Design review of the part built by this model. Coordinates are the model's own, in mm. A direction names the side the tool comes from. Round coordinates to 2 decimals unless told otherwise and drop trailing zeros. Order: outer loops, then holes, each group sorted by start corner. A loop starts at its lowest first (then second) coordinate and runs counter-clockwise, first axis right, second up. Notation, with made-up numbers: (16, 14.5) - (33, 14.5) arc R31 ccw to (33, 46.5) - close; hole circle Ø2 at (33, -15.75). An arc over 180 degrees is marked (long way). Use CSV: the item, a comma, the result in double quotes.
from build123d import *

# Parameters (mm, degrees)
SKETCH1_W              = 200
SKETCH1_H              = 140
BOSS_EXTRUDE1_DEPTH    = 6.35
SKETCH4_W              = 65
SKETCH4_H              = 6.35
BOSS_EXTRUDE2_DEPTH    = 6.35
LPATTERN1_COUNT        = 2
LPATTERN1_PITCH        = 85
SKETCH5_W              = 6.35
SKETCH5_H              = 65
BOSS_EXTRUDE3_DEPTH    = 6.35
SKETCH6_W              = 65
SKETCH6_H              = 6.35
CUT_EXTRUDE3_DEPTH     = 6.35
SKETCH7_R              = 2
CUT_EXTRUDE4_DEPTH     = 6.35
FILLET4_R              = 1
LPATTERN2_COUNT        = 2
LPATTERN2_PITCH        = 85
FILLET4_OF_LPATTERN2_R = 1
FILLET5_R              = 5
SKETCH8_R              = 2
CUT_EXTRUDE6_DEPTH     = 6.35
FILLET6_R              = 1


with BuildPart() as part:
    # Sketch1 → Boss-Extrude1 (new body)
    with BuildSketch(Plane(origin=(0, 0, 0), x_dir=(1, 0, 0), z_dir=(0, 1, 0))):
        Rectangle(SKETCH1_W, SKETCH1_H)
    extrude(amount=-BOSS_EXTRUDE1_DEPTH)

    # Sketch4 → Boss-Extrude2 (add)
    with BuildSketch(Plane(origin=(0, 0, 0), x_dir=(1, 0, 0), z_dir=(0, 1, 0))):
        with Locations((-42.5, -73.175)):
            Rectangle(SKETCH4_W, SKETCH4_H)
    boss_extrude2 = extrude(amount=-BOSS_EXTRUDE2_DEPTH)

    # LPattern1: Boss-Extrude2 ×2
    with Locations(*[(i * LPATTERN1_PITCH, 0, 0) for i in range(1, LPATTERN1_COUNT)]):
        add(boss_extrude2)

    # Sketch5 → Boss-Extrude3 (add)
    with BuildSketch(Plane(origin=(0, 0, 0), x_dir=(1, 0, 0), z_dir=(0, 1, 0))):
        with Locations((-103.175, 0)):
            Rectangle(SKETCH5_W, SKETCH5_H)
    extrude(amount=-BOSS_EXTRUDE3_DEPTH)

    # Sketch6 → Cut-Extrude3 (cut)
    with BuildSketch(Plane(origin=(0, 0, 0), x_dir=(1, 0, 0), z_dir=(0, 1, 0))):
        with Locations((42.5, 58.425)):
            Rectangle(SKETCH6_W, SKETCH6_H)
    cut_extrude3 = extrude(amount=-CUT_EXTRUDE3_DEPTH, mode=Mode.SUBTRACT)

    # Sketch7 → Cut-Extrude4 (cut)
    with BuildSketch(Plane(origin=(0, 0, 0), x_dir=(1, 0, 0), z_dir=(0, 1, 0))):
        with Locations((10, 55.25)):
            Circle(SKETCH7_R)
        with Locations((75, 55.25)):
            Circle(SKETCH7_R)
        with Locations((10, 61.6)):
            Circle(SKETCH7_R)
        with Locations((75, 61.6)):
            Circle(SKETCH7_R)
    cut_extrude4 = extrude(amount=-CUT_EXTRUDE4_DEPTH, mode=Mode.SUBTRACT)

    # Fillet4
    fillet4_edges = [part.edges().sort_by_distance(p)[0] for p in [
        (73, -3.175, -55.25),
        (12, -3.175, -55.25),
        (75, -3.175, -59.6),
        (12, -3.175, -61.6),
        (10, -3.175, -57.25),
        (73, -3.175, -61.6),
        (75, -3.175, -57.25),
        (10, -3.175, -59.6),
    ]]
    fillet(fillet4_edges, radius=FILLET4_R)

    # LPattern2: Cut-Extrude3, Cut-Extrude4 ×2
    with Locations(*[(-i * LPATTERN2_PITCH, 0, 0) for i in range(1, LPATTERN2_COUNT)]):
        add(cut_extrude3, mode=Mode.SUBTRACT)
        add(cut_extrude4, mode=Mode.SUBTRACT)

    # Fillet4 of LPattern2
    fillet4_of_lpattern2_edges = [part.edges().sort_by_distance(p)[0] for p in [
        (-12, -3.175, -55.25),
        (-73, -3.175, -55.25),
        (-10, -3.175, -59.6),
        (-73, -3.175, -61.6),
        (-75, -3.175, -57.25),
        (-12, -3.175, -61.6),
        (-10, -3.175, -57.25),
        (-75, -3.175, -59.6),
    ]]
    fillet(fillet4_of_lpattern2_edges, radius=FILLET4_OF_LPATTERN2_R)

    # Fillet5
    fillet5_edges = [part.edges().sort_by_distance(p)[0] for p in [
        (100, -3.175, 70),
        (-100, -3.175, 70),
        (-100, -3.175, -70),
        (100, -3.175, -70),
    ]]
    fillet(fillet5_edges, radius=FILLET5_R)

    # Sketch8 → Cut-Extrude6 (cut)
    with BuildSketch(Plane(origin=(0, 0, 0), x_dir=(1, 0, 0), z_dir=(0, 1, 0))):
        with Locations((-75, -70)):
            Circle(SKETCH8_R)
        with Locations((-10, -70)):
            Circle(SKETCH8_R)
        with Locations((10, -70)):
            Circle(SKETCH8_R)
        with Locations((75, -70)):
            Circle(SKETCH8_R)
        with Locations((-100, 32.5)):
            Circle(SKETCH8_R)
        with Locations((-100, -32.5)):
            Circle(SKETCH8_R)
    extrude(amount=-CUT_EXTRUDE6_DEPTH, mode=Mode.SUBTRACT)

    # Fillet6
    fillet6_edges = [part.edges().sort_by_distance(p)[0] for p in [
        (-75, -3.175, 76.35),
        (-10, -3.175, 76.35),
        (10, -3.175, 76.35),
        (75, -3.175, 76.35),
        (-102, -3.175, -32.5),
        (-102, -3.175, 32.5),
        (75, -3.175, 72),
        (10, -3.175, 72),
        (-10, -3.175, 72),
        (-75, -3.175, 72),
        (-100, -3.175, -34.5),
        (77, -3.175, 70),
        (8, -3.175, 70),
        (-8, -3.175, 70),
        (-100, -3.175, 34.5),
        (-77, -3.175, 70),
        (-106.35, -3.175, 32.5),
        (-106.35, -3.175, -32.5),
    ]]
    fillet(fillet6_edges, radius=FILLET6_R)


solid = part.part
1) Insertion check: pin 1 Ø1.3 at (y, z) = (-2.5, 74.5) entering from +X; pin 2 Ø0.8 at (y, z) = (-1.5, 74) entering from -X; pin 3 Ø3 at (y, z) = (-4.5, 51) entering from -X. Each pin has a flat end and moves straight along its axis. Give the tip position at first contact, or say it passes through.
Data:
pin 1,"stops at x = 75"
pin 2,"stops at x = -75"
pin 3,"stops at x = -100"
2) For faces 4 (the face through (-87, -3, 70)), 5 (the face through (-43, -3, -61.6)), 6 (the face through (-100, -3, -50)), list the 3-axis set-ups (+Z, -Z, +X, -X, +Y, -Y) from which the entire face can be reached by the end or side of a thin tool; tool diameter is ignored.
Data:
face 4,"+Z, -X, +Y, -Y"
face 5,"+Y, -Y"
face 6,"-Z, -X, +Y, -Y"
3) To check wall thickness, follow L1, parallel to Z at x = -59, y = -4; L2, parallel to Z at x = 74.5, y = -3.5; L3, parallel to Z at x = -82, y = -4.5. State the ranges of each line that lie inside material, in increasing order. Write a range as from..to.
Data:
L1,"z = -70..-61.6, -55.25..76.35"
L2,"z = -70..-63.54, -53.31..68.06, 71.96..76.22"
L3,"z = -70..70"
4) We need section B-B (y = -2.75). Give the number of separate pieces and of enclosed holes in the cut face, then the cut area to 3 significant figures.
Data:
separate pieces,"1"
enclosed holes,"2"
area,"28,300 mm2"
5) The part is to be moulded in two halves that separate along Z. For faces 1 (the face through (-11.374, -3.131, 68.546)), 2 (the face through (-43, -3, 76.35)), 3 (the face through (-5, 0, 2)), say which applies: +Z half, -Z half, draft (parallel to the pull), parting line (faces both ways), or undercut.
Data:
face 1,"undercut"
face 2,"+Z half"
face 3,"draft"
6) We need section C-C (x = -89). Give the boundary of the cut face in (y, z).
Data:
outline,"(-6.35, -70) - (0, -70) - (0, 70) - (-6.35, 70) - close"
7) We need section A-A (x = 66). Give the boundary of the cut face in (y, z).
Data:
outline,"(-6.35, -70) - (0, -70) - (0, -61.6) - (-6.35, -61.6) - close; (-6.35, -55.25) - (0, -55.25) - (0, 76.35) - (-6.35, 76.35) - close"
